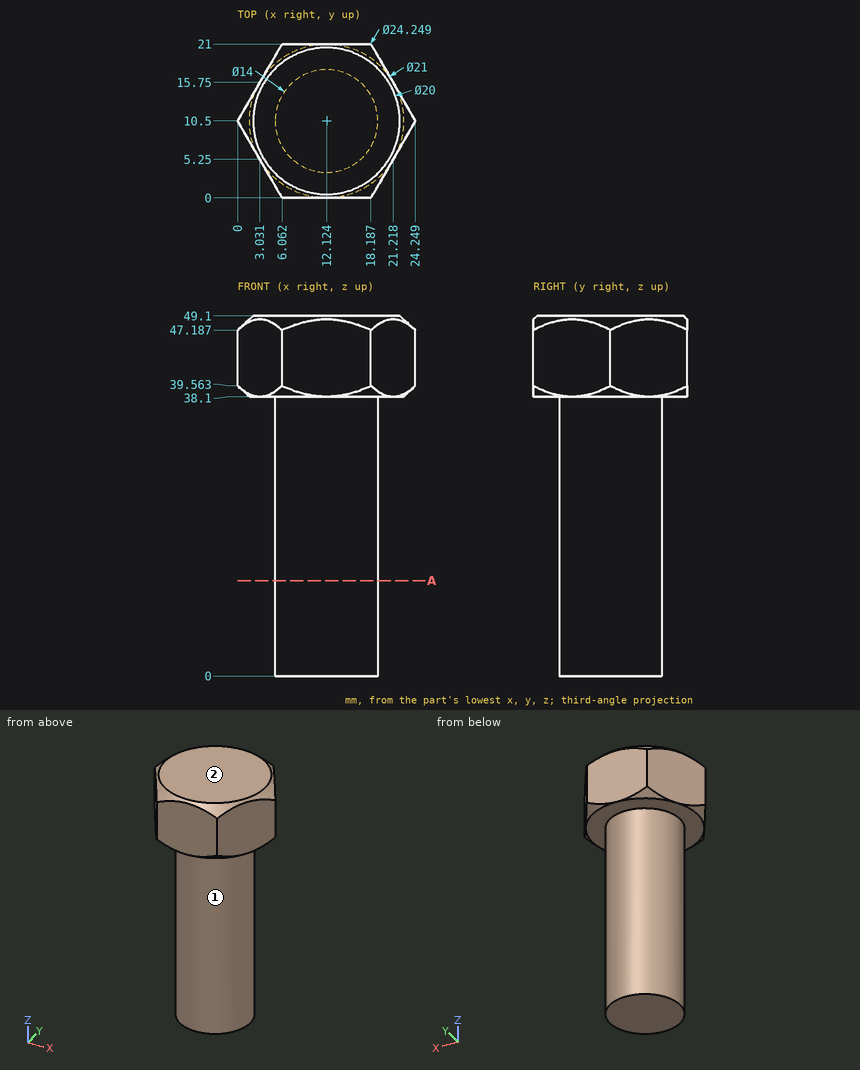
Verification items for this drawing (mm, ordinates from the low corner). A direction names the side the tool comes from. Round coordinates to 2 decimals unless told otherwise and drop trailing zeros. Order: outer loops, then holes, each group sorted by start corner. A loop starts at its lowest first (then second) coordinate and runs counter-clockwise, first axis right, second up. Notation, with made-up numbers: (-12.75, -11.75) - (-7.75, -11.75) arc R29 cw to (-7.75, 10.25) - close; hole circle Ø6 at (21.25, 19.5). An arc over 180 degrees is marked (long way). Use CSV: the item, a comma, the result in double quotes. Start each with the question number.
1) Access from +Z, -Z, +X, -X, +Y, -Y to the whole of each face (thin tool, end or side, straight path). Record for the marked faces 1 and 2.
2) Go/stop test with flat-tipped pins: P1, Ø8, axis at x = 13.5, z = 9, coming from the +Y side; P2, Ø12, axis at x = 17, z = 7.5, coming from the -Y side; P3, Ø6, axis at y = 6.5, z = 38.5, coming from the -X side. Record where each tip stops, or that it passes through.
3) Section check A-A, the plane z = 13. Record the cut outline in (x, y) (1 decimal), plus the area to 3 significant figures.
4) Thickness scan on L1, parallel to Z at x = 10, y = 3; L2, parallel to X at y = 16, z = 31.5 (1 decimal); L3, parallel to X at y = 11, z = 35. Record the ranges inside material, lowest first.
Answers:
1,face 1,"-Z"
1,face 2,"+Z, +X, -X, +Y, -Y"
2,P1,"stops at y = 17.5"
2,P2,"stops at y = 3.5"
2,P3,"stops at x = 0.61"
3,outline,"circle Ø14 at (12.1, 10.5)"
3,area,"154 mm²"
4,L1,"z = 38.1 to 49.1"
4,L2,"x = 7.8 to 16.5"
4,L3,"x = 5.14 to 19.11"
